Autodesk Inventor part; units mm, degrees
ref_plane "YZ Plane" through (0, 0, 0) normal (1, 0, 0) x (0, 1, 0)
ref_plane "XZ Plane" through (0, 0, 0) normal (0, 1, 0) x (-1, 0, 0)
ref_plane "XY Plane" through (0, 0, 0) normal (0, 0, 1) x (1, 0, 0)
sketch "Sketch1" plane through (0, 0, 0) normal (0, 1, 0) x (-1, 0, 0)
  arc A0 (-15, 27) -> (-13, 25) centre (-13, 27) ccw
  line L0 (-15, 27) -> (-15, 53)
  arc A1 (-13, 55) -> (-15, 53) centre (-13, 53) ccw
  line L1 (-13, 55) -> (13, 55)
  arc A2 (15, 53) -> (13, 55) centre (13, 53) ccw
  line L2 (15, 53) -> (15, 27)
  arc A3 (13, 25) -> (15, 27) centre (13, 27) ccw
  line L3 (13, 25) -> (-13, 25)
  arc A4 (36.5, 1.5) -> (38.5, 3.5) centre (36.5, 3.5) ccw
  line L4 (38.5, 3.5) -> (38.5, 76.5)
  arc A5 (38.5, 76.5) -> (36.5, 78.5) centre (36.5, 76.5) ccw
  line L5 (36.5, 78.5) -> (-36.5, 78.5)
  arc A6 (-36.5, 78.5) -> (-38.5, 76.5) centre (-36.5, 76.5) ccw
  line L6 (-38.5, 76.5) -> (-38.5, 3.5)
  arc A7 (-38.5, 3.5) -> (-36.5, 1.5) centre (-36.5, 3.5) ccw
  line L7 (-36.5, 1.5) -> (36.5, 1.5)
  circle A8 centre (0, 60) radius 2.5
  circle A9 centre (-10, 70) radius 2.5
  circle A10 centre (10, 70) radius 2.5
  circle A11 centre (30, 70) radius 2.75
  circle A12 centre (10, 10) radius 2.5
  circle A13 centre (30, 10) radius 2.75
  circle A14 centre (0, 20) radius 2.5
  circle A15 centre (20, 30) radius 2.5
  circle A16 centre (20, 60) radius 2.5
  circle A17 centre (20, 50) radius 2.5
  circle A18 centre (-20, 30) radius 2.5
  circle A19 centre (-30, 40) radius 2.75
  circle A20 centre (-20, 20) radius 2.5
  circle A21 centre (20, 20) radius 2.5
  circle A22 centre (-20, 60) radius 2.5
  circle A23 centre (-10, 10) radius 2.5
  circle A24 centre (-30, 10) radius 2.75
  circle A25 centre (-30, 70) radius 2.75
  circle A26 centre (30, 40) radius 2.75
  circle A27 centre (-20, 50) radius 2.5
  line L8 (13, 53) -> (-13, 27)
  line L9 (-13, 53) -> (13, 27)
  line L10 (0, 0) -> (0, 40)
  line L11 (0, 0) -> (0, -40)
  line L12 (36.4941, 78.5) -> (-36.5, 78.5)
  line L13 (-38.5, 78.5) -> (-38.5, -56.3967)
  line L14 (-36.5, -66.5) -> (36.4941, -66.5)
  line L15 (38.4941, -59.5) -> (38.4941, 76.5)
  arc A28 (38.4941, 76.5) -> (36.4941, 78.5) centre (36.4941, 76.5) ccw
  arc A29 (-36.5, 78.5) -> (-38.5, 76.5) centre (-36.5, 76.5) ccw
  arc A30 (-38.5, -56.3967) -> (-36.5, -58.3967) centre (-36.5, -56.3967) ccw
  arc A31 (36.4941, -66.5) -> (38.4941, -64.5) centre (36.4941, -64.5) ccw
  line L16 (-38.5, -59.5) -> (-38.5, -56.3967)
  arc A32 (-38.5, -64.5) -> (-36.5, -66.5) centre (-36.5, -64.5) ccw
  circle A33 centre (0, -35) radius 20
  arc A34 (-25.4017, -7.1967) -> (-28.4017, -10.1967) centre (-25.4017, -10.1967) ccw
  line L17 (-28.4017, -10.1967) -> (-28.4017, -61.3967)
  arc A35 (-28.4017, -61.3967) -> (-26.4017, -63.3967) centre (-26.4017, -61.3967) ccw
  line L18 (-26.4017, -63.3967) -> (24.7983, -63.3967)
  arc A36 (24.7983, -63.3967) -> (27.7983, -60.3967) centre (24.7983, -60.3967) ccw
  line L19 (27.7983, -60.3967) -> (27.7983, -10.1967)
  arc A37 (27.7983, -10.1967) -> (24.7983, -7.1967) centre (24.7983, -10.1967) ccw
  line L20 (24.7983, -7.1967) -> (-25.4017, -7.1967)
  circle A38 centre (23.2983, -11.6967) radius 2.75
  circle A39 centre (-23.9017, -11.6967) radius 2.75
  circle A40 centre (23.2983, -58.8967) radius 2.75
  circle A41 centre (-23.9017, -58.8967) radius 2.75
  line L21 (38.4941, -59.5) -> (38.4941, -64.5)
  line L22 (-38.5, -64.5) -> (-38.5, -59.5)
  line L23 (-10, 40) -> (11.2302, 40)
  line L24 (0, 80) -> (0, 40)
  line L25 (0, 80) -> (0, 120)
  line L26 (-38.5, 1.5) -> (-38.5, 136.3967)
  line L27 (-36.5, 146.5) -> (36.4941, 146.5)
  line L28 (38.4941, 139.5) -> (38.4941, 3.5)
  arc A42 (-36.5, 138.3967) -> (-38.5, 136.3967) centre (-36.5, 136.3967) ccw
  arc A43 (38.4941, 144.5) -> (36.4941, 146.5) centre (36.4941, 144.5) ccw
  line L29 (-38.5, 139.5) -> (-38.5, 136.3967)
  arc A44 (-36.5, 146.5) -> (-38.5, 144.5) centre (-36.5, 144.5) ccw
  circle A45 centre (0, 115) radius 20
  arc A46 (-28.4017, 90.1967) -> (-25.4017, 87.1967) centre (-25.4017, 90.1967) ccw
  line L30 (-28.4017, 90.1967) -> (-28.4017, 141.3967)
  arc A47 (-26.4017, 143.3967) -> (-28.4017, 141.3967) centre (-26.4017, 141.3967) ccw
  line L31 (-26.4017, 143.3967) -> (24.7983, 143.3967)
  arc A48 (27.7983, 140.3967) -> (24.7983, 143.3967) centre (24.7983, 140.3967) ccw
  line L32 (27.7983, 140.3967) -> (27.7983, 90.1967)
  arc A49 (24.7983, 87.1967) -> (27.7983, 90.1967) centre (24.7983, 90.1967) ccw
  line L33 (24.7983, 87.1967) -> (-25.4017, 87.1967)
  circle A50 centre (23.2983, 91.6967) radius 2.75
  circle A51 centre (-23.9017, 91.6967) radius 2.75
  circle A52 centre (23.2983, 138.8967) radius 2.75
  circle A53 centre (-23.9017, 138.8967) radius 2.75
  line L34 (38.4941, 139.5) -> (38.4941, 144.5)
  line L35 (-38.5, 144.5) -> (-38.5, 139.5)
  point P0 (-38.5, 1.5)
  point P1 (0, 40)
  point P2 (-38.5, -61.5)
  point P3 (36.4941, 78.5)
  point P4 (38.4941, 3.3463)
  point P5 (36.5, 78.5)
  point P6 (0, 1.5)
  point P7 (36.4941, 78.5)
  point P8 (36.4941, -66.5)
  point P9 (-38.5, 141.5)
  point P10 (38.4941, 76.6537)
  point P11 (36.4941, 146.5)
  dimension "d0" = 40
  dimension "d1" = 40
  dimension "d2" = 2
  dimension "d5" = 145
  dimension "d6" = 0
  dimension "d7" = 2
  dimension "d13" = 5.5
  dimension "d14" = 5.5
  dimension "d15" = 5.5
  dimension "d16" = 5.5
  dimension "d17" = 5.5
  dimension "d18" = 5.5
  dimension "d20" = 40
  dimension "d21" = 5.5
  dimension "d22" = 5.5
  dimension "d23" = 5.5
  dimension "d24" = 5.5
extrude "Extrusion1" add sketch "Sketch1" along normal blind 10 contours A0 L3 L10 A14 L7 A7 L6 A6 L5 L24 A8 L1 A1 L0 | L3 A3 L2 A2 L1 L24 A8 L5 A28 L15 A4 L7 L10 A14 | L10 A14 | A14 L10 | L24 A8 | A8 L24 | L7 A4 L15 L21 A31 L14 A32 L22 L16 L13 A7 | L20 A37 L19 A36 L18 A35 L17 A34 | L5 A6 L13 L26 L29 L35 A44 L27 A43 L34 L28 A5 | L33 A46 L30 A47 L31 A48 L32 A49 | A9 | A10 | A12 | A15 | A16 | A17 | A18 | A20 | A21 | A22 | A23 | A27
sketch "Sketch3" plane through (0, 10, 0) normal (0, 1, 0) x (1, 0, 0)
  line L0 (15, -27) -> (15, -53)
  arc A0 (15, -27) -> (13, -25) centre (13, -27) ccw
  line L1 (-13, -25) -> (13, -25)
  arc A1 (-13, -25) -> (-15, -27) centre (-13, -27) ccw
  line L2 (-15, -53) -> (-15, -27)
  line L3 (13, -55) -> (-13, -55)
  arc A2 (13, -55) -> (15, -53) centre (13, -53) ccw
  arc A3 (-15, -53) -> (-13, -55) centre (-13, -53) ccw
  point P0 (0, 0)
extrude "Extrusion2" add sketch "Sketch3" against normal blind 10
sketch "Sketch5" plane through (0, 10, 0) normal (0, 1, 0) x (1, 0, 0)
  circle A0 centre (-23.2983, 11.6967) radius 2.75
  line L0 (8.6601, 21.3463) -> (-11.3399, 21.3463)
  line L1 (8.6601, 51.3463) -> (8.6601, 21.3463)
  line L2 (8.6601, 21.3463) -> (-11.3399, 21.3463)
  arc A1 (-21.3399, 31.3463) -> (-11.3399, 21.3463) centre (-11.3399, 31.3463) ccw
  line L3 (-21.3399, 31.3463) -> (-21.3399, 41.3463)
  arc A2 (-11.3399, 51.3463) -> (-21.3399, 41.3463) centre (-11.3399, 41.3463) ccw
  line L4 (-11.3399, 51.3463) -> (8.6601, 51.3463)
  circle A3 centre (23.9017, 11.6967) radius 2.75
  circle A4 centre (23.9017, 58.8967) radius 2.75
  circle A5 centre (-23.2983, 11.6967) radius 2.75
  circle A6 centre (-23.2983, 58.8967) radius 2.75
  line L5 (37.0974, 65.5992) -> (-35.8967, 65.5992)
  arc A7 (-35.8967, 65.5992) -> (-37.8967, 63.5992) centre (-35.8967, 63.5992) ccw
  line L6 (-37.8967, 63.5992) -> (-37.8967, 6.0933)
  line L7 (-37.8967, 6.0933) -> (-37.8967, 3.0933)
  line L8 (39.0974, 3.0933) -> (-37.8967, 3.0933)
  line L9 (39.0974, 63.5992) -> (39.0974, 3.0933)
  arc A8 (39.0974, 63.5992) -> (37.0974, 65.5992) centre (37.0974, 63.5992) ccw
  circle A9 centre (-23.2983, 11.6967) radius 2.75
  point P0 (0, 0)
  point P1 (0.6033, 35.5933)
  point P2 (-11.3399, 21.3463)
sketch "Sketch6" plane through (0, 10, 0) normal (0, 1, 0) x (1, 0, 0)
  circle A0 centre (0, 35) radius 20
  point P0 (0, 0)
extrude "Extrusion3" add sketch "Sketch6" against normal up to surface (10 mm away)
extrude "Extrusion4" cut sketch "Sketch5" against normal blind 10 contours L0 A1 L3 A2 L4 L1
sketch "Sketch7" plane through (-38.4941, 0, 76.6537) normal (-1, 0, 0) x (0, 0, 1)
  line L0 (67.8463, 10) -> (-141.1537, 10)
  line L1 (67.8463, 0) -> (-141.1537, 0)
  line L2 (2.4973, 10) -> (-2.5509, 10)
  line L3 (-2.5509, 10) -> (-2.5509, 0)
  line L4 (-2.5509, 0) -> (2.4973, 0)
  line L5 (2.4973, 0) -> (2.4973, 10)
  point P0 (-76.6537, 0)
extrude "Extrusion5" add sketch "Sketch7" against normal blind 4
sketch "Sketch8" plane through (0, 10, 0) normal (0, 1, 0) x (1, 0, 0)
  line L0 (-38.4941, 64.5) -> (-38.4941, -144.5)
  line L1 (-38.4941, 0) -> (43.0425, 0)
  line L2 (43.0425, 0) -> (43.0425, 71.8354)
  line L3 (43.0425, 71.8354) -> (-38.4941, 71.8354)
  line L4 (-38.4941, 71.8354) -> (-38.4941, 0)
  point P0 (0, 0)
extrude "Extrusion6" cut sketch "Sketch8" against normal through all
fillet "Fillet1" radius 2 2 edges at (38.5, 5, 0) (-38.4941, 5, 0)
properties part number "afirma_motor_lado"
Here's how the part is built. I have some questions about the finished solid (model axes, mm). Coordinates: 2 decimals unless noted, no trailing zeros. Order: outer loops, then holes, each group sorted by start corner. A loop starts at its lowest first (then second) coordinate and runs counter-clockwise, first axis right, second up. Notation, with made-up numbers: (49, 88.25) - (67, 88.25) arc R18 cw to (67, 94.25) - close; hole circle Ø4 at (20, 38.5). An arc over 180 degrees is marked (long way). Use CSV: the item, a comma, the result in double quotes. Start each with the question number.
1. Suppose I cut it at C-C on z = 125. List the corners of the cut face in (x, y) for me, then the cut area to 3 significant figures.
2. Suppose I cut it at D-D on x = 0. List the corners of the cut face in (y, z) for me, then the cut area to 4 significant figures.
3. If we mould it in two halves opening along Z, with no side actions, what happens to faces 1 (the face through (-1, 5, 0)), 2 (the face through (32.027, 4.93, 68.141)), 3 (the face through (38.5, 5, 74))? For each: +Z half, -Z half, draft (parallel to the pull), parting line (faces both ways), or undercut.
4. Suppose I cut it at A-A on x = -30. List the corners of the cut face in (y, z) for me, then the cut area to 3 significant figures.
5. Suppose I cut it at B-B on z = 10. List the corners of the cut face in (x, y) for me, then the cut area to 3 significant figures.
6. Please list where these lines run through material, in increasing order: line 1 (Z direction, x = -30, y = 4.75); line 2 (X direction, y = 2, z = 137.5); line 3 (Z direction, x = -25, y = 8). Write a range as from..to.
Output:
1,outline,"(-38.49, 0) - (-17.32, 0) - (-17.32, 10) - (-38.49, 10) - close; (17.32, 0) - (38.5, 0) - (38.5, 10) - (17.32, 10) - close"
1,area,"424 mm2"
2,outline,"(0, 0) - (10, 0) - (10, 95) - (0, 95) - close; (0, 135) - (10, 135) - (10, 146.5) - (0, 146.5) - close"
2,area,"1,065 mm2"
3,face 1,"-Z half"
3,face 2,"undercut"
3,face 3,"draft"
4,outline,"(0, 0) - (10, 0) - (10, 7.25) - (0, 7.25) - close; (0, 12.75) - (10, 12.75) - (10, 37.25) - (0, 37.25) - close; (0, 42.75) - (10, 42.75) - (10, 67.25) - (0, 67.25) - close; (0, 72.75) - (10, 72.75) - (10, 146.5) - (0, 146.5) - close"
4,area,"1,300 mm2"
5,outline,"(-38.49, 0) - (-32.75, 0) - (-32.75, 10) - (-38.49, 10) - close; (-27.25, 0) - (27.25, 0) - (27.25, 10) - (-27.25, 10) - close; (32.75, 0) - (38.5, 0) - (38.5, 10) - (32.75, 10) - close"
5,area,"660 mm2"
6,line 1,"z = 0..7.25, 12.75..37.25, 42.75..67.25, 72.75..146.5"
6,line 2,"x = -38.49..-25.67, -20.93..21.53, 26.27..38.5"
6,line 3,"z = 0..89.54, 93.86..136.74, 141.06..146.5"
